Check sheet for the modelled part. Datum: model origin and axes. Units: mm. Round coordinates to 2 decimals unless told otherwise and drop trailing zeros. Loops run counter-clockwise (first coordinate to the right, second up) from the corner with the lowest first, then second, coordinate; pieces in that order, holes last. Notation, with made-up numbers: (-13.75, -10) - (1.25, -10) arc R16 ccw to (1.25, 12) - close; hole circle Ø11 at (30.5, 34). An arc over 180 degrees is marked (long way). Put each result on its own line as item: value. Start each with the question number.
Item 1: Section check D-D, the plane y = 5.25. Record the cut outline in (x, z).
Item 2: Material ranges on line 1 along Y through (x, z) = (8, 0); line 2 along Z through (x, y) = (2.5, 1.75), recorded low to high.
Item 3: Section check C-C, the plane z = 0. Record the cut outline in (x, y).
Item 4: Section check B-B, the plane x = -2.75. Record the cut outline in (y, z).
Item 5: Gauge pin test, flat ends, axial feed: pin 1 Ø2 at (x, y) = (3.5, -6) entering from -Z; pin 2 Ø10 at (x, z) = (15, -5.5) entering from +Y; pin 3 Ø1 at (y, z) = (-2, -3.5) entering from +X. Record the tip position at first contact, or that the pin passes through.
Item 6: Section check A-A, the plane y = 0. Record the cut outline in (x, z).
from build123d import *

# Parameters (mm, degrees)
SKETCH_1_R      = 10
SKETCH_1_R_2    = 8.5
EXTRUDE_1_DEPTH = 20
EXTRUDE_7_DEPTH = 5
EXTRUDE_START   = 5
SKETCH_4_R      = 10
SKETCH_4_R_2    = 8.5
EXTRUDE_8_DEPTH = 5


with BuildPart() as part:
    # Sketch 1 → Extrude 1 (new body)
    with BuildSketch(Plane(origin=(0, 0, 0), x_dir=(0, 0, -1), z_dir=(1, 0, 0))):
        Circle(SKETCH_1_R)
        Circle(SKETCH_1_R_2, mode=Mode.SUBTRACT)
    extrude(amount=EXTRUDE_1_DEPTH)



with BuildPart() as body_2:
    # Sketch 2 → Extrude 7 (new body)
    with BuildSketch(Plane.ZY):
        with BuildLine():
            ThreePointArc((8.5, 0), (4.563441684, 7.171122646), (-3.6, 7.7))
            Line((-3.6, 7.7), (-3.6, 0))
            Line((-3.6, 0), (-3.6, -7.7))
            ThreePointArc((-3.6, -7.7), (4.563441684, -7.171122646), (8.5, 0))
        make_face()
    extrude(amount=EXTRUDE_7_DEPTH)


with BuildPart() as part_1:
    add(part.part)

    add(body_2.part)  # Extrude 8 merges body 2
    # Sketch 4 → Extrude 8 (add)
    with BuildSketch(Plane.ZY.offset(EXTRUDE_START)):
        Circle(SKETCH_4_R)
        with Locations(Location((0, 0, 0), (0, 0, 244.942384582))):
            Circle(SKETCH_4_R_2, mode=Mode.SUBTRACT)
    extrude(amount=-EXTRUDE_8_DEPTH)


solid = part_1.part
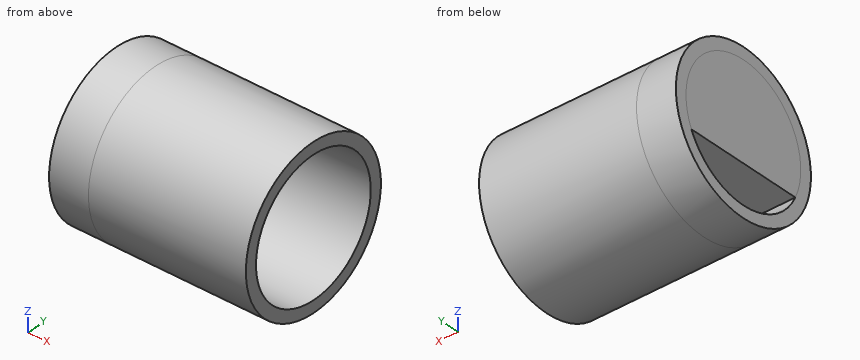
Check result:
1. outline: (-5, -8.51) - (20, -8.51) - (20, -6.68) - (-5, -6.68) - close; (-5, -3.6) - (0, -3.6) - (0, 6.68) - (20, 6.68) - (20, 8.51) - (-5, 8.51) - close
2. line 1: -10 to -8.5, 8.5 to 10
2. line 2: -9.85 to -8.32, 8.32 to 9.85
3. outline: (-5, -10) - (20, -10) - (20, -8.5) - (0, -8.5) - (0, 8.5) - (20, 8.5) - (20, 10) - (-5, 10) - close
4. outline: circle Ø20 at (0, 0); hole (-7.7, -3.6) arc R8.5 ccw to (7.7, -3.6) - close
5. pin 1: z = -8.66
5. pin 2: y = 9.99
5. pin 3: x = 0
6. outline: (-5, -10) - (20, -10) - (20, -8.5) - (-5, -8.5) - close; (-5, -3.6) - (0, -3.6) - (0, 8.5) - (20, 8.5) - (20, 10) - (-5, 10) - close
